Read the model definition and answer for the solid it produces. Units are mm, in the model's axes. Face numbers are marked on the shaded views. A direction names the side the tool comes from. Coordinates: 2 decimals unless noted, no trailing zeros. Write each loop counter-clockwise with the first axis right and the second up, starting at its lowest first coordinate (ties: lowest second). Pieces come first, ordered by that corner, then holes. Notation, with made-up numbers: (-20, 26) - (13, 26) arc R20 cw to (13, 57) - close; hole circle Ø1 at (25, -23.75). An arc over 180 degrees is marked (long way). Return JSON: item names as keys, results as strings.
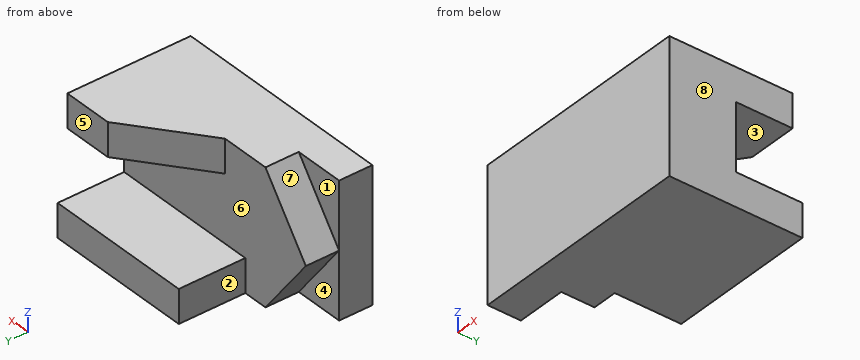
```python
from build123d import *

# Parameters (mm, degrees)
SKETCH1_W           = 13.5
SKETCH1_H           = 8
BOSS_EXTRUDE1_DEPTH = 2
BOSS_EXTRUDE2_DEPTH = 2
SKETCH3_W           = 9
SKETCH3_H           = 2
SKETCH3_W_2         = 7.5
BOSS_EXTRUDE3_DEPTH = 4
CUT_EXTRUDE1_DEPTH  = 4


with BuildPart() as part:
    # Sketch1 → Boss-Extrude1 (new body)
    with BuildSketch(Plane(origin=(0, 0, 0), x_dir=(1, 0, 0), z_dir=(0, 1, 0))):
        Rectangle(SKETCH1_W, SKETCH1_H)
    extrude(amount=BOSS_EXTRUDE1_DEPTH)

    # Sketch2 → Boss-Extrude2 (add)
    with BuildSketch(Plane(origin=(0, 2, 0), x_dir=(1, 0, 0), z_dir=(0, 1, 0))):
        Polygon((-6.75, 0), (-3.75, 4), (6.75, 4), (6.75, -4), (-3.75, -4), align=None)
    extrude(amount=BOSS_EXTRUDE2_DEPTH)

    # Sketch3 → Boss-Extrude3 (add)
    with BuildSketch(Plane(origin=(0, 4, 0), x_dir=(1, 0, 0), z_dir=(0, 1, 0))):
        with Locations((2.25, 3)):
            Rectangle(SKETCH3_W, SKETCH3_H)
        with Locations((3, -3)):
            Rectangle(SKETCH3_W_2, SKETCH3_H)
    extrude(amount=BOSS_EXTRUDE3_DEPTH)

    # Sketch4 → Cut-Extrude1 (cut)
    with BuildSketch(Plane.XY.offset(4)):
        Polygon((6.75, 7.413398543), (3.75, 7.413398543), (-0.75, 4), (-0.75, 8), (6.75, 8), align=None)
    extrude(amount=-CUT_EXTRUDE1_DEPTH, mode=Mode.SUBTRACT)


solid = part.part
```
(1) A cutting plane is placed at B-B (x = 5.75). Determine the outline of the cut face in (y, z).
Answer:
{"outline": "(0, -4) - (8, -4) - (8, -2) - (4, -2) - (4, 2) - (7.41, 2) - (7.41, 4) - (0, 4) - close"}
(2) Which of the six approach directions +Z, -Z, +X, -X, +Y, -Y give full straight-line access (tool end or side, diameter ignored) to the marked faces 1, 2, 3, 4 and 5?
Answer:
{"face 1": "+Z, -X, +Y", "face 2": "+Z, -Z, -X, +Y", "face 3": "+X, -X, +Y", "face 4": "-Z, -X, +Y", "face 5": "+Z, +X, -X, +Y"}
(3) Straight lines are drawn through the part: line 1 (Z direction, x = 5.75, y = 6.25); line 2 (X direction, y = 7.25, z = -3.5); line 3 (Y direction, x = 5.25, z = 2.75). For each, find the intervals that lie inside material, in ascending order. Write a range as from..to.
Answer:
{"line 1": "-4..-2, 2..4", "line 2": "-2.25..6.75", "line 3": "0..7.41"}
(4) A cutting plane is placed at C-C (z = -3.5). Determine the outline of the cut face in (x, y) (3 decimals), and give its area (4 significant figures).
Answer:
{"outline": "(-6.75, 0) - (6.75, 0) - (6.75, 8) - (-2.25, 8) - (-2.25, 4) - (-4.125, 4) - (-4.125, 2) - (-6.75, 2) - close", "area": "84.75 mm²"}
(5) A cutting plane is placed at D-D (y = 3). Determine the outline of the cut face in (x, z), and give its area (3 significant figures).
Answer:
{"outline": "(-6.75, 0) - (-3.75, -4) - (6.75, -4) - (6.75, 4) - (-3.75, 4) - close", "area": "96.0 mm²"}
(6) Determine the mould class of the marked faces 6, 7 and 8 for opening direction Z: +Z half, -Z half, draft (parallel to the pull), parting line (faces both ways), or undercut.
Answer:
{"face 6": "undercut", "face 7": "+Z half", "face 8": "draft"}
(7) Flat-ended cylindrical pins translate along their axes: P1, Ø1.6, axis at x = 4.5, z = 2.5, coming from the +Y side; P2, Ø0.6, axis at y = 6, z = -3, coming from the -X side; P3, Ø0.9, axis at x = -5, z = 2.5, coming from the +Y side. Find the tip coordinate at first contact, or state that the pin passes through.
Answer:
{"P1": "y = 7.41", "P2": "x = -2.25", "P3": "y = 4"}
(8) A cutting plane is placed at A-A (y = 6.25). Determine the outline of the cut face in (x, z), and give its area (3 significant figures).
Answer:
{"outline": "(-2.25, -4) - (6.75, -4) - (6.75, -2) - (-2.25, -2) - close; (2.22, 2) - (6.75, 2) - (6.75, 4) - (2.22, 4) - close", "area": "27.1 mm²"}
